Input: part model. Units: mm. Frame: model coordinates. Give positions to 0.01 mm unless a question says otherwise; leave off trailing zeros. Loops run counter-clockwise (first coordinate to the right, second up) from the corner with the lowest first, then second, coordinate; pieces in that order, holes last. Notation, with made-up numbers: (42.25, 17) - (47.25, 17) arc R18 cw to (47.25, 49) - close; hole circle Ø3 at (-14.5, 37.5). An arc over 180 degrees is marked (long way). Answer as a JSON object with one key per item and string values. Group by question number.
(1) Section query B-B (x = 32). Return loops of the section in (y, z), plus the area to 3 significant figures.
(2) Section query A-A (z = -44). Return loops of the section in (x, y), plus the area to 3 significant figures.
(3) Material intervals for L1, parallel to Z at x = 27.5, y = 0.7; L2, parallel to X at y = 1.2, z = -59.5; L3, parallel to Z at x = -63, y = 1.35, sorted ascending.
(4) Mould query, pull axis Z, two halves, no side actions, for faces 1 (the cylindrical face through (-15.777, 1.014, -6.841)), 2 (the flat face through (-30, 0, -20)). Classes: +Z half, -Z half, draft (parallel to the pull), parting line (faces both ways), or undercut.
(5) Section query C-C (z = 14). Return loops of the section in (x, y).
(6) Section query D-D (y = 0.75). Count the separate pieces of the cut face and the enclosed holes in it, plus the area to 3 significant figures.
(7) Pin query (flat end, axial travel): P1, Ø1.7, axis at x = -75.48, z = -35.43, coming from the -Y side. Return the tip coordinate at first contact, or that it passes through.
```python
from build123d import *

# Parameters (mm, degrees)
SKETCH1_W              = 180
SKETCH1_H              = 120
BOSS_EXTRUDE1_DEPTH    = 2
BUTTON_HOLES_CUT_REACH = 144.444
SKETCH2_R              = 14.2
SKETCH2_R_2            = 12
SKETCH2_R_3            = 20.01
M2_5_CLEARANCE_HOLE1_D = 2.9


with BuildPart() as part:
    # Sketch1 → Boss-Extrude1 (new body)
    with BuildSketch(Plane(origin=(0, 0, 0), x_dir=(1, 0, 0), z_dir=(0, 1, 0))):
        with Locations((-28.728476821, 18.675496689)):
            Rectangle(SKETCH1_W, SKETCH1_H)
    extrude(amount=BOSS_EXTRUDE1_DEPTH)

    # Sketch2 → button_holes_cut (cut, up to next)
    with BuildSketch(Plane(origin=(0, 2, 0), x_dir=(1, 0, 0), z_dir=(0, 1, 0)), mode=Mode.PRIVATE) as button_holes_cut_sk1:
        with Locations(Location((-50.338026535, -20.041382951, 0), (0, 0, 270))):
            Circle(SKETCH2_R)
    button_holes_cut_tool1 = extrude(button_holes_cut_sk1.sketch, amount=-BUTTON_HOLES_CUT_REACH, mode=Mode.PRIVATE) & part.part
    # Sketch2 → button_holes_cut (cut, up to next)
    with BuildSketch(Plane(origin=(0, 2, 0), x_dir=(1, 0, 0), z_dir=(0, 1, 0)), mode=Mode.PRIVATE) as button_holes_cut_sk2:
        with Locations(Location((29.661973465, 59.958617049, 0), (0, 0, 270))):
            Circle(SKETCH2_R_2)
    button_holes_cut_tool2 = extrude(button_holes_cut_sk2.sketch, amount=-BUTTON_HOLES_CUT_REACH, mode=Mode.PRIVATE) & part.part
    # Sketch2 → button_holes_cut (cut, up to next)
    with BuildSketch(Plane(origin=(0, 2, 0), x_dir=(1, 0, 0), z_dir=(0, 1, 0)), mode=Mode.PRIVATE) as button_holes_cut_sk3:
        with Locations(Location((-10.338026535, 59.958617049, 0), (0, 0, 270))):
            Circle(SKETCH2_R_2)
    button_holes_cut_tool3 = extrude(button_holes_cut_sk3.sketch, amount=-BUTTON_HOLES_CUT_REACH, mode=Mode.PRIVATE) & part.part
    # Sketch2 → button_holes_cut (cut, up to next)
    with BuildSketch(Plane(origin=(0, 2, 0), x_dir=(1, 0, 0), z_dir=(0, 1, 0)), mode=Mode.PRIVATE) as button_holes_cut_sk4:
        with Locations(Location((-10.338026535, -20.041382951, 0), (0, 0, 270))):
            Circle(SKETCH2_R)
    button_holes_cut_tool4 = extrude(button_holes_cut_sk4.sketch, amount=-BUTTON_HOLES_CUT_REACH, mode=Mode.PRIVATE) & part.part
    # Sketch2 → button_holes_cut (cut, up to next)
    with BuildSketch(Plane(origin=(0, 2, 0), x_dir=(1, 0, 0), z_dir=(0, 1, 0)), mode=Mode.PRIVATE) as button_holes_cut_sk5:
        with Locations(Location((29.661973465, -20.041382951, 0), (0, 0, 270))):
            Circle(SKETCH2_R)
    button_holes_cut_tool5 = extrude(button_holes_cut_sk5.sketch, amount=-BUTTON_HOLES_CUT_REACH, mode=Mode.PRIVATE) & part.part
    # Sketch2 → button_holes_cut (cut, up to next)
    with BuildSketch(Plane(origin=(0, 2, 0), x_dir=(1, 0, 0), z_dir=(0, 1, 0)), mode=Mode.PRIVATE) as button_holes_cut_sk6:
        with Locations(Location((-50.338026535, 19.958617049, 0), (0, 0, 270))):
            Circle(SKETCH2_R)
    button_holes_cut_tool6 = extrude(button_holes_cut_sk6.sketch, amount=-BUTTON_HOLES_CUT_REACH, mode=Mode.PRIVATE) & part.part
    # Sketch2 → button_holes_cut (cut, up to next)
    with BuildSketch(Plane(origin=(0, 2, 0), x_dir=(1, 0, 0), z_dir=(0, 1, 0)), mode=Mode.PRIVATE) as button_holes_cut_sk7:
        with Locations(Location((-10.338026535, 19.958617049, 0), (0, 0, 270))):
            Circle(SKETCH2_R)
    button_holes_cut_tool7 = extrude(button_holes_cut_sk7.sketch, amount=-BUTTON_HOLES_CUT_REACH, mode=Mode.PRIVATE) & part.part
    # Sketch2 → button_holes_cut (cut, up to next)
    with BuildSketch(Plane(origin=(0, 2, 0), x_dir=(1, 0, 0), z_dir=(0, 1, 0)), mode=Mode.PRIVATE) as button_holes_cut_sk8:
        with Locations(Location((29.661973465, 19.958617049, 0), (0, 0, 270))):
            Circle(SKETCH2_R)
    button_holes_cut_tool8 = extrude(button_holes_cut_sk8.sketch, amount=-BUTTON_HOLES_CUT_REACH, mode=Mode.PRIVATE) & part.part
    # Sketch2 → button_holes_cut (cut, up to next)
    with BuildSketch(Plane(origin=(0, 2, 0), x_dir=(1, 0, 0), z_dir=(0, 1, 0)), mode=Mode.PRIVATE) as button_holes_cut_sk9:
        with Locations(Location((-91.728476821, 51.675496689, 0), (0, 0, 270))):
            Circle(SKETCH2_R_3)
    button_holes_cut_tool9 = extrude(button_holes_cut_sk9.sketch, amount=-BUTTON_HOLES_CUT_REACH, mode=Mode.PRIVATE) & part.part
    add(button_holes_cut_tool1.solids().sort_by_distance((-50.338027, 2, 20.041383))[0], mode=Mode.SUBTRACT)
    add(button_holes_cut_tool2.solids().sort_by_distance((29.661973, 2, -59.958617))[0], mode=Mode.SUBTRACT)
    add(button_holes_cut_tool3.solids().sort_by_distance((-10.338027, 2, -59.958617))[0], mode=Mode.SUBTRACT)
    add(button_holes_cut_tool4.solids().sort_by_distance((-10.338027, 2, 20.041383))[0], mode=Mode.SUBTRACT)
    add(button_holes_cut_tool5.solids().sort_by_distance((29.661973, 2, 20.041383))[0], mode=Mode.SUBTRACT)
    add(button_holes_cut_tool6.solids().sort_by_distance((-50.338027, 2, -19.958617))[0], mode=Mode.SUBTRACT)
    add(button_holes_cut_tool7.solids().sort_by_distance((-10.338027, 2, -19.958617))[0], mode=Mode.SUBTRACT)
    add(button_holes_cut_tool8.solids().sort_by_distance((29.661973, 2, -19.958617))[0], mode=Mode.SUBTRACT)
    add(button_holes_cut_tool9.solids().sort_by_distance((-91.728477, 2, -51.675497))[0], mode=Mode.SUBTRACT)

    # M2.5 Clearance Hole1 (through all)
    with Locations(Plane(origin=(0, 2, 0), x_dir=(1, 0, 0), z_dir=(0, 1, 0))):
        with Locations((-91.728476821, 51.675496689), (-75.478476821, 67.925496689), (-107.978476821, 67.925496689), (-75.478476821, 35.425496689), (-107.978476821, 35.425496689)):
            Hole(M2_5_CLEARANCE_HOLE1_D / 2)


solid = part.part
```
Recorded:
{
 "1": {"outline": "(0, -78.68) - (2, -78.68) - (2, -71.73) - (0, -71.73) - close; (0, -48.19) - (2, -48.19) - (2, -33.96) - (0, -33.96) - close; (0, -5.95) - (2, -5.95) - (2, 6.04) - (0, 6.04) - close; (0, 34.05) - (2, 34.05) - (2, 41.32) - (0, 41.32) - close", "area": "80.9 mm^2"},
 "2": {"outline": "(-118.73, 0) - (-110.21, 0) - (-110.21, 2) - (-118.73, 2) - close; (-73.25, 0) - (61.27, 0) - (61.27, 2) - (-73.25, 2) - close", "area": "286 mm^2"},
 "3": {"L1": "z = -78.68 to -71.76, -48.15 to -33.99, -5.92 to 6.01, 34.08 to 41.32", "L2": "x = -118.73 to -110.15, -73.31 to -22.33, 1.65 to 17.67, 41.65 to 61.27", "L3": "z = -78.68 to -26.39, -13.53 to 13.61, 26.47 to 41.32"},
 "4": {"face 1": "undercut", "face 2": "draft"},
 "5": {"outline": "(-118.73, 0) - (-63.19, 0) - (-63.19, 2) - (-118.73, 2) - close; (-37.49, 0) - (-23.19, 0) - (-23.19, 2) - (-37.49, 2) - close; (2.51, 0) - (16.81, 0) - (16.81, 2) - (2.51, 2) - close; (42.51, 0) - (61.27, 0) - (61.27, 2) - (42.51, 2) - close"},
 "6": {"separate pieces": "1", "enclosed holes": "13", "area": "15,600 mm^2"},
 "7": {"P1": "passes through"}
}
